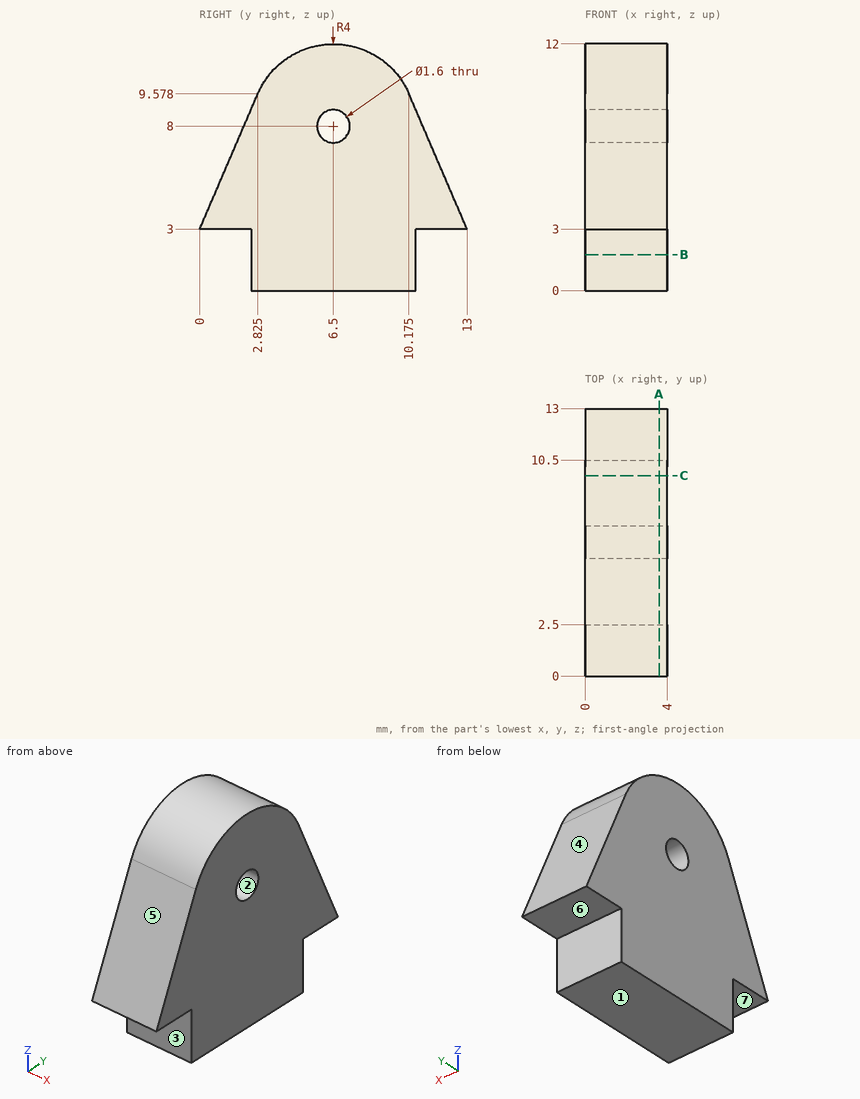
Answer from the drawing. Dimensions are ordinates in mm from the lowest x, y and z of the part. A direction names the side the tool comes from. Coordinates: 2 decimals unless noted, no trailing zeros. Write each loop counter-clockwise with the first axis right and the second up, starting at its lowest first coordinate (ties: lowest second). Pieces come first, ordered by that corner, then holes. Notation, with made-up numbers: M 13.25,43.25 L 48.25,43.25 A22 ccw 48.25,53.25 Z; hole C -12.5,69.25 d10. An arc over 180 degrees is marked long. Put each result on its own line as item: value. Start each with the question number.
1. A cutting plane is placed at C-C on y = 9.75. Write down the section's boundary in (x, z).
2. Which of the six approach directions +Z, -Z, +X, -X, +Y, -Y give full straight-line access (tool end or side, diameter ignored) to the marked faces 5, 6 and 7?
3. A cutting plane is placed at A-A on x = 3.6. Write down the section's boundary in (y, z) (1 decimal).
4. For a pull along Y with two mould halves and no side action, classify the marked faces 1, 2, 3 and 4 as pulls with the +Y half, pulls with the -Y half, needs draft (parallel to the pull), parting line crosses it, or undercut.
5. Consider line 1 (Z direction, x = 0.85, y = 6.5); line 2 (Y direction, x = 3.65, z = 1); line 3 (Y direction, x = 3.6, z = 7.5) (1 decimal). Determine where each line is inside the solid, lowest interval first. Write a range as from..to.
6. Flat-ended cylindrical pins translate along their axes: P1, Ø1, axis at x = 3, y = 10, coming from the +Z side (1 decimal); P2, Ø1.5, axis at x = 2.5, z = 1, coming from the -Y side; P3, Ø1.5, axis at x = 2.5, z = 2, coming from the +Y side. Find the tip coordinate at first contact, or state that the pin passes through.
7. A cutting plane is placed at B-B on z = 1.75. Write down the section's boundary in (x, y).
Resolved:
1. outline: M 0,0 L 4,0 L 4,10.33 L 0,10.33 Z
2. face 5: +Z, +X, -X, -Y
2. face 6: -Z, +X, -X, +Y
2. face 7: -Z, +X, -X, -Y
3. outline: M 0,3 L 2.5,3 L 2.5,0 L 10.5,0 L 10.5,3 L 13,3 L 10.2,9.6 A4 ccw 2.8,9.6 Z; hole C 6.5,8 d1.6
4. face 1: needs draft
4. face 2: undercut
4. face 3: pulls with the -Y half
4. face 4: pulls with the +Y half
5. line 1: z = 0..7.2, 8.8..12
5. line 2: y = 2.5..10.5
5. line 3: y = 1.9..5.9, 7.1..11.1
6. P1: stops at z = 10.6
6. P2: stops at y = 2.5
6. P3: stops at y = 10.5
7. outline: M 0,2.5 L 4,2.5 L 4,10.5 L 0,10.5 Z
